from build123d import *

# Parameters (mm, degrees)
F1_DEPTH = 30
F3_D     = 2.5
F5_D     = 2.5
F5_DEPTH = 21
F5_TIP   = 0.7510757738
F6_R     = 3
F7_R     = 2.5
F8_DEPTH = 60.001
F9_R     = 3


with BuildPart() as f1:
    # F0 (on Top) → F1 (new body, symmetric)
    with BuildSketch(Plane.XY):
        Polygon((-20, 21), (-28, 21), (-28, -21), (28, -21), (28, 21), (20, 21), (20, 1), (-20, 1), align=None)
    extrude(amount=F1_DEPTH, both=True)

    # F3 (through all)
    with Locations(Plane(origin=(-28, 0, 0), x_dir=(0, -1, 0), z_dir=(-1, 0, 0))):
        with Locations((-11, 20), (-11, -20)):
            Hole(F3_D / 2)

    # F5
    with Locations(Plane.XZ.offset(21)):
        with Locations((0, 20), (-21, -20), (21, -20)):
            Hole(F5_D / 2, depth=F5_DEPTH)
            with Locations((0, 0, -(F5_DEPTH + F5_TIP / 2))):  # 118° drill point
                Cone(0, F5_D / 2, F5_TIP, mode=Mode.SUBTRACT)

    # F6
    f6_edges = [f1.edges().sort_by_distance(p)[0] for p in [
        (-28, -21, 0),
        (28, -21, 0),
        (-28, 21, 0),
        (-20, 21, 0),
        (20, 21, 0),
        (28, 21, 0),
    ]]
    fillet(f6_edges, radius=F6_R)

    # F7 (on face) → F8 (cut, through all)
    with BuildSketch(Plane.XY.offset(30)):
        with Locations((-20, 1)):
            Circle(F7_R)
        with Locations((20, 1)):
            Circle(F7_R)
    extrude(amount=-F8_DEPTH, mode=Mode.SUBTRACT)

    # F9
    f9_edges = [f1.edges().sort_by_distance(p)[0] for p in [
        (-17.5, 1, 0),
        (-20, 3.5, 0),
        (17.5, 1, 0),
        (20, 3.5, 0),
    ]]
    fillet(f9_edges, radius=F9_R)


solid = f1.part
Model file for the job. Use its own axes, mm. A direction names the side the tool comes from. Give positions to 0.01 mm unless a question says otherwise; leave off trailing zeros. Loops run counter-clockwise (first coordinate to the right, second up) from the corner with the lowest first, then second, coordinate; pieces in that order, holes last. Notation, with made-up numbers: (5.25, -16.5) -> (52.25, -16.5) arc R24 cw to (52.25, 22.5) -> close; hole circle Ø7 at (16.25, 29). An arc over 180 degrees is marked (long way). Use a Markdown table: item, result. Add a question column.
(1) Slice it at B-B on z = 12.5. List the corners of the cut face in (x, y).
(2) Tool access for faces 1 (the flat face through (28, 0, 0)), 2 (the cylindrical face through (20.373, 4.161, 0.42)), 3 (the cylindrical face through (-20.9, 20.14, -0.42)), 4 (the cylindrical face through (22.25, -10.4, -19.95)): list every direction of +Z, -Z, +X, -X, +Y, -Y with a clear straight run to the whole face (end or side of a thin tool).
(3) Drop flat-ended pins along their axis: pin 1 Ø10 at (x, y) = (4.5, 3.5) entering from +Z; pin 2 Ø2 at (x, z) = (21, -20) entering from -Y; pin 3 Ø1.5 at (x, z) = (0, 20) entering from +Y. Give the stop position or say it passes through.
(4) Mould opens along Z. For faces 5 (the flat face through (0, -4, -30)), 6 (the flat face through (0, -21, 0)), 7 (the cylindrical face through (-23.94, 10.01, -20.76)) say: +Z half, -Z half, draft (parallel to the pull), parting line (faces both ways), or undercut.
(5) Slice it at D-D on x = 19. List the corners of the cut face in (y, z), and give its area (3 significant figures).
(6) Wall check: line 1 along X through (y, z) = (-12, -20); line 2 along Z through (x, y) = (-26, 11); line 3 along X through (y, z) = (16, 0). Give the ranges that are in metal, low to high.
(7) Slice it at C-C on x = -3. List the corners of the cut face in (y, z), and give its area (3 significant figures).
(8) Slice it at A-A on y = 7.5. List the corners of the cut face in (x, z).
Filled sheet:
| question | item | result |
|---|---|---|
| 1 | outline | (-28, -18) arc R3 ccw to (-25, -21) -> (25, -21) arc R3 ccw to (28, -18) -> (28, 18) arc R3 ccw to (25, 21) -> (23, 21) arc R3 ccw to (20, 18) -> (20, 5.61) arc R3 ccw to (21.36, 3.1) arc R2.5 cw (long way) to (17.9, -0.36) arc R3 ccw to (15.39, 1) -> (-15.39, 1) arc R3 ccw to (-17.9, -0.36) arc R2.5 cw (long way) to (-21.36, 3.1) arc R3 ccw to (-20, 5.61) -> (-20, 18) arc R3 ccw to (-23, 21) -> (-25, 21) arc R3 ccw to (-28, 18) -> close |
| 2 | face 1 | +Z, -Z, +X, +Y, -Y |
| 2 | face 2 | +Z, -Z |
| 2 | face 3 | +Z, -Z, +Y |
| 2 | face 4 | -Y |
| 3 | pin 1 | z = 30 |
| 3 | pin 2 | y = 2.5 |
| 3 | pin 3 | y = 1 |
| 4 | face 5 | -Z half |
| 4 | face 6 | draft |
| 4 | face 7 | undercut |
| 5 | outline | (-21, -30) -> (-1.29, -30) -> (-1.29, 30) -> (-21, 30) -> close |
| 5 | area | 1,180 mm2 |
| 6 | line 1 | -28 to -22.25, -19.75 to 19.75, 22.25 to 28 |
| 6 | line 2 | -30 to -21.25, -18.75 to 18.75, 21.25 to 30 |
| 6 | line 3 | -28 to -20, 20 to 28 |
| 7 | outline | (-21, -30) -> (1, -30) -> (1, 30) -> (-21, 30) -> close |
| 7 | area | 1,320 mm2 |
| 8 | outline | (-28, -30) -> (-20, -30) -> (-20, 30) -> (-28, 30) -> close; (20, -30) -> (28, -30) -> (28, 30) -> (20, 30) -> close |
